Geometry check sheet. Reference: drawing and pictorial views, mm from the part's lowest x, y, z. Give positions to 0.01 mm unless a question says otherwise; leave off trailing zeros. Write each loop counter-clockwise with the first axis right and the second up, starting at its lowest first coordinate (ties: lowest second). Pieces come first, ordered by that corner, then holes. Notation, with made-up numbers: M 27.25,-7 L 85.25,-7 A18 ccw 85.25,22 Z; hole C -27,88 d8. An arc over 180 degrees is marked long. Answer as a JSON object with one key per item and string values.
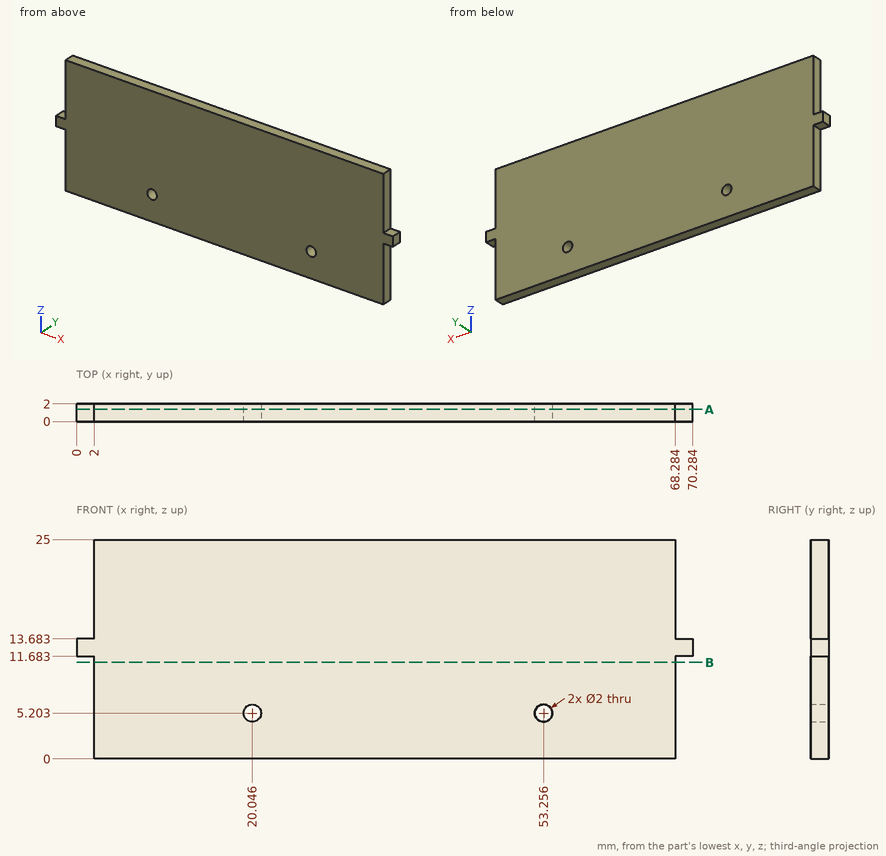
1) Section check A-A on y = 1.4. Record the boundary of the cut face in (x, z) (1 decimal), and give its area (3 significant figures).
Completed:
{"outline": "M 0,11.7 L 2,11.7 L 2,0 L 68.3,0 L 68.3,11.7 L 70.3,11.7 L 70.3,13.7 L 68.3,13.7 L 68.3,25 L 2,25 L 2,13.7 L 0,13.7 Z; hole C 20,5.2 d2; hole C 53.3,5.2 d2", "area": "1,660 mm2"}
2) Section check B-B on z = 11. Record the boundary of the cut face in (x, y) (1 decimal).
Completed:
{"outline": "M 2,0 L 68.3,0 L 68.3,2 L 2,2 Z"}
3) Thickness scan on L1, parallel to X at y = 1.35, z = 3.75 (1 decimal); L2, parallel to Z at x = 54, y = 1.05 (1 decimal). Record the ranges inside material, lowest first.
Completed:
{"L1": "x = 2 to 68.3", "L2": "z = 0 to 4.5, 5.9 to 25"}
4) Go/stop test with flat-tipped pins: pin 1 (1 mm diameter, centred on x = 1, y = 1.5, fed in from -Z); pin 2 (1 mm diameter, centred on x = 69.5, y = 1, fed in from +Z). Record where each tip stops, or that it passes through.
Completed:
{"pin 1": "stops at z = 11.68", "pin 2": "stops at z = 13.68"}
